For this review, take the finished solid that the model builds, in its own axes (mm). A direction names the side the tool comes from. Round coordinates to 2 decimals unless told otherwise and drop trailing zeros. Loops run counter-clockwise (first coordinate to the right, second up) from the corner with the lowest first, then second, coordinate; pieces in that order, holes last. Notation, with made-up numbers: (66.25, 34.25) -> (120.25, 34.25) arc R27 cw to (120.25, 50.25) -> close; hole circle Ø7 at (-13, 32.5). An arc over 180 degrees is marked (long way). Write each question's results on one line, items separated by ' | '.
```python
from build123d import *

# Parameters (mm, degrees)
SKETCH1_W           = 390
SKETCH1_H           = 382.5
SKETCH1_R           = 90
BOSS_EXTRUDE1_DEPTH = 12
SKETCH2_W           = 472.5
SKETCH2_H           = 105
SKETCH2_W_2         = 120
SKETCH2_H_2         = 45
SKETCH2_W_3         = 105
BOSS_EXTRUDE2_DEPTH = 90
BOSS_EXTRUDE3_DEPTH = 90
CUT_EXTRUDE1_DEPTH  = 90


with BuildPart() as part:
    # Sketch1 → Boss-Extrude1 (new body)
    with BuildSketch(Plane.XY):
        Rectangle(SKETCH1_W, SKETCH1_H)
        with Locations((0, 26.25)):
            Circle(SKETCH1_R, mode=Mode.SUBTRACT)
    extrude(amount=BOSS_EXTRUDE1_DEPTH)

    # Sketch2 → Boss-Extrude2 (add)
    with BuildSketch(Plane.XY.offset(12)):
        with Locations((0, -243.75)):
            Rectangle(SKETCH2_W, SKETCH2_H)
        with Locations((135, -243.75)):
            Rectangle(SKETCH2_W_2, SKETCH2_H_2, mode=Mode.SUBTRACT)
        with Locations((0, -243.75)):
            Rectangle(SKETCH2_W_3, SKETCH2_H_2, mode=Mode.SUBTRACT)
        with Locations((-135, -243.75)):
            Rectangle(SKETCH2_W_2, SKETCH2_H_2, mode=Mode.SUBTRACT)
    extrude(amount=-BOSS_EXTRUDE2_DEPTH)

    # Sketch3 → Boss-Extrude3 (add)
    with BuildSketch(Plane(origin=(0, -191.25, 0), x_dir=(1, 0, 0), z_dir=(0, 1, 0))):
        Polygon((195, -12), (236.25, 50.637349082), (230.737913281, 54.267349082), (195, 0), align=None)
    boss_extrude3 = extrude(amount=BOSS_EXTRUDE3_DEPTH)

    # Sketch4 → Cut-Extrude1 (cut)
    with BuildSketch(Plane(origin=(141.524586719, 0, 93.201409187), x_dir=(0.5500000000000003, 0, -0.8351646544245032), z_dir=(0.8351646544245033, 0, 0.5500000000000003))):
        Polygon((172.228024147, -101.25), (107.25, -101.25), (172.228024147, -191.25), align=None)
    cut_extrude1 = extrude(amount=-CUT_EXTRUDE1_DEPTH, mode=Mode.SUBTRACT)

    # Mirror1: Boss-Extrude3, Cut-Extrude1 across plane
    add(boss_extrude3.mirror(Plane(origin=(0, 0, 0), x_dir=(0, 0, 1), z_dir=(1, 0, 0))))
    add(cut_extrude1.mirror(Plane(origin=(0, 0, 0), x_dir=(0, 0, 1), z_dir=(1, 0, 0))), mode=Mode.SUBTRACT)


solid = part.part
```
1. Consider section D-D (y = -256.5). State the section outline as (x, z) points, plus the area to 3 significant figures.
Values found:
outline: (-236.25, -78) -> (-195, -78) -> (-195, 12) -> (-236.25, 12) -> close; (-75, -78) -> (-52.5, -78) -> (-52.5, 12) -> (-75, 12) -> close; (52.5, -78) -> (75, -78) -> (75, 12) -> (52.5, 12) -> close; (195, -78) -> (236.25, -78) -> (236.25, 12) -> (195, 12) -> close | area: 11,500 mm2
2. Consider section B-B (y = 7). State the section outline as (x, z) points, plus the area to 3 significant figures.
Values found:
outline: (-195, 0) -> (-87.92, 0) -> (-87.92, 12) -> (-195, 12) -> close; (87.92, 0) -> (195, 0) -> (195, 12) -> (87.92, 12) -> close | area: 2,570 mm2
3. Consider section A-A (x = 0). State the section outline as (y, z) points.
Values found:
outline: (-296.25, -78) -> (-266.25, -78) -> (-266.25, 12) -> (-296.25, 12) -> close; (-221.25, -78) -> (-191.25, -78) -> (-191.25, 0) -> (-63.75, 0) -> (-63.75, 12) -> (-221.25, 12) -> close; (116.25, 0) -> (191.25, 0) -> (191.25, 12) -> (116.25, 12) -> close
4. To check wall thickness, follow probe 1 along Y at (x, z) = (0, 7.25); probe 2 along Y at (x, z) = (-125, -13); probe 3 along X at (y, z) = (26, 6). State the ranges of each line that lie inside material, in increasing order.
Values found:
probe 1: y = -296.25 to -266.25, -221.25 to -63.75, 116.25 to 191.25 | probe 2: y = -296.25 to -266.25, -221.25 to -191.25 | probe 3: x = -195 to -90, 90 to 195
5. For pin 1 (20.5 mm diameter, centred on x = -214.5, z = -26, fed in from +Y); pin 2 (3 mm diameter, centred on x = -88.5, y = 21, fed in from -Z); pin 3 (6 mm diameter, centred on y = 37, z = 4, fed in from +X), all flat-tipped, find the tip position at first contact; note any pin that passes through.
Values found:
pin 1: stops at y = -131.98 | pin 2: stops at z = 0 | pin 3: stops at x = 195
6. Draft analysis for pull direction Y (two halves, no side actions). For faces 1 (the face through (-136, -221.25, -32)), 2 (the face through (215.413, -145.62, -24.913)), 3 (the face through (-3, -296.25, -32)), state which applies: released by +Y, released by -Y, zero draft, split by the parting line, or undercut.
Values found:
face 1: undercut | face 2: released by +Y | face 3: released by -Y
7. Tool access review of faces 4 (the face through (-3, -82, 0)), 5 (the face through (210.753, -156.88, -11.921)), 6 (the face through (-1, -221.25, -32)): name each direction out of +Z, -Z, +X, -X, +Y, -Y from which nothing blocks a thin tool from reaching the whole face with its end or side.
Values found:
face 4: -Z, +Y | face 5: +Z, +X, +Y | face 6: +Z, -Z
8. Consider section C-C (x = -116). State the section outline as (y, z) points, plus the area to 3 significant figures.
Values found:
outline: (-296.25, -78) -> (-266.25, -78) -> (-266.25, 12) -> (-296.25, 12) -> close; (-221.25, -78) -> (-191.25, -78) -> (-191.25, 0) -> (191.25, 0) -> (191.25, 12) -> (-221.25, 12) -> close | area: 9,990 mm2
